Design review of the part built by this model. Coordinates are the model's own, in mm. A direction names the side the tool comes from. Give positions to 0.01 mm unless a question says otherwise; leave off trailing zeros. Order: outer loops, then holes, each group sorted by start corner. A loop starts at its lowest first (then second) coordinate and runs counter-clockwise, first axis right, second up. Notation, with made-up numbers: (5, -7.5) -> (41, -7.5) arc R29 ccw to (41, 26.5) -> close; hole circle Ø4 at (49.5, 50.25). An arc over 180 degrees is marked (long way). Use a Markdown table: item, result. Add a question column.
```python
from build123d import *

# Parameters (mm, degrees)
ESQUISSE1_W             = 70
ESQUISSE1_H             = 62
ESQUISSE1_R             = 2.25
BOSS_EXTRU_3_DEPTH      = 6
ESQUISSE3_W             = 70
ESQUISSE3_H             = 5.5
BOSS_EXTRU_4_DEPTH      = 50
ESQUISSE4_R             = 1.1
ENL_V_MAT_EXTRU_1_DEPTH = 88.550819181
ESQUISSE5_R             = 5
ENL_V_MAT_EXTRU_2_DEPTH = 50


with BuildPart() as part:
    # Esquisse1 → Boss.-Extru.3 (new body)
    with BuildSketch(Plane.XY):
        with Locations((1.563587615, -10.397163121)):
            Rectangle(ESQUISSE1_W, ESQUISSE1_H)
        with Locations((-13.036412385, 6.752836879)):
            Circle(ESQUISSE1_R, mode=Mode.SUBTRACT)
        with Locations((16.163587615, 6.752836879)):
            Circle(ESQUISSE1_R, mode=Mode.SUBTRACT)
        with Locations((-13.036412385, -21.247163121)):
            Circle(ESQUISSE1_R, mode=Mode.SUBTRACT)
        with Locations((16.163587615, -21.247163121)):
            Circle(ESQUISSE1_R, mode=Mode.SUBTRACT)
    extrude(amount=BOSS_EXTRU_3_DEPTH)

    # Esquisse3 → Boss.-Extru.4 (add)
    with BuildSketch(Plane.XY.offset(6)):
        with Locations((1.563587615, -38.647163121)):
            Rectangle(ESQUISSE3_W, ESQUISSE3_H)
    extrude(amount=BOSS_EXTRU_4_DEPTH)

    # Esquisse4 → Enlèv. mat.-Extru.1 (cut, through all)
    with BuildSketch(Plane(origin=(0, -35.897163121, 0), x_dir=(1, 0, 0), z_dir=(0, 1, 0))):
        with Locations(Location((-6.886412385, -32.194360359, 0), (0, 0, 270))):
            Circle(ESQUISSE4_R)
        with Locations(Location((5.613587615, -32.194360359, 0), (0, 0, 270))):
            Circle(ESQUISSE4_R)
    extrude(amount=-ENL_V_MAT_EXTRU_1_DEPTH, mode=Mode.SUBTRACT)

    # Esquisse5 → Enlèv. mat.-Extru.2 (cut)
    with BuildSketch(Plane(origin=(0, 0, 0), x_dir=(-1, 0, 0), z_dir=(0, 0, -1))):
        with Locations((-1.563587615, 8.602836879)):
            Circle(ESQUISSE5_R)
    extrude(amount=-ENL_V_MAT_EXTRU_2_DEPTH, mode=Mode.SUBTRACT)


solid = part.part
```
1) The part is to be moulded in two halves that separate along X. For faces 1 (the flat face through (36.564, -24, 5)), 2 (the flat face through (-33.436, -24, 5)), 3 (the flat face through (1, 20.603, 3)), 4 (the cylindrical face through (14.38, 5.38, 2.96)), say which applies: +X half, -X half, draft (parallel to the pull), parting line (faces both ways), or undercut.
2) Add section C-C (x = -2.5). Give the boundary of the cut face in (y, z), then the cut area to 3 significant figures.
3) Add section A-A (x = 15). Give the boundary of the cut face in (y, z).
4) Insertion check: pin 1 (2 mm diameter, centred on x = -15.5, z = 35.5, fed in from +Y); pin 2 (5 mm diameter, centred on x = -13.04, y = 6.75, fed in from +Z). Each pin has a flat end and moves straight along its axis. Give the tip position at first contact, or say it passes through.
5) Add section D-D (y = -34.5). Give the boundary of the cut face in (x, z).
6) Machinability: for faces 5 (the flat face through (1, -41.397, 28)), 6 (the flat face through (1, -7, 6)), which of the approach directions +Z, -Z, +X, -X, +Y, -Y give a long, thin tool a straight path to every point of the face, cutting with its end or side? Answer none if there is none.
7) Add section B-B (y = -20). Give the boundary of the cut face in (x, z), then the cut area to 3 significant figures.
8) For L1, parallel to Y at x = 32.5, z = 31.5; L2, parallel to Z at x = -23, y = -30; L3, parallel to X at y = 8.5, z = 3, list the stretches that pass through material, from the lowest coordinate up. Write a range as [from, to].
Worked answers:
| question | item | result |
|---|---|---|
| 1 | face 1 | +X half |
| 1 | face 2 | -X half |
| 1 | face 3 | draft |
| 1 | face 4 | undercut |
| 2 | outline | (-41.4, 0) -> (5.69, 0) -> (5.69, 6) -> (-35.9, 6) -> (-35.9, 56) -> (-41.4, 56) -> close; (11.52, 0) -> (20.6, 0) -> (20.6, 6) -> (11.52, 6) -> close |
| 2 | area | 612 mm^2 |
| 3 | outline | (-41.4, 0) -> (-23.17, 0) -> (-23.17, 6) -> (-35.9, 6) -> (-35.9, 56) -> (-41.4, 56) -> close; (-19.32, 0) -> (4.83, 0) -> (4.83, 6) -> (-19.32, 6) -> close; (8.68, 0) -> (20.6, 0) -> (20.6, 6) -> (8.68, 6) -> close |
| 4 | pin 1 | y = -35.9 |
| 4 | pin 2 | z = 6 |
| 5 | outline | (-33.44, 0) -> (36.56, 0) -> (36.56, 6) -> (-33.44, 6) -> close |
| 6 | face 5 | +Z, -Z, +X, -X, -Y |
| 6 | face 6 | +Z, +X, -X, +Y |
| 7 | outline | (-33.44, 0) -> (-14.91, 0) -> (-14.91, 6) -> (-33.44, 6) -> close; (-11.16, 0) -> (14.29, 0) -> (14.29, 6) -> (-11.16, 6) -> close; (18.04, 0) -> (36.56, 0) -> (36.56, 6) -> (18.04, 6) -> close |
| 7 | area | 375 mm^2 |
| 8 | L1 | [-41.4, -35.9] |
| 8 | L2 | [0, 6] |
| 8 | L3 | [-33.44, -14.45], [-11.62, -3.44], [6.56, 14.75], [17.58, 36.56] |
